Read the model definition and answer for the solid it produces. Units are mm, in the model's axes. A direction names the side the tool comes from. Coordinates: 2 decimals unless noted, no trailing zeros. Write each loop counter-clockwise with the first axis right and the second up, starting at its lowest first coordinate (ties: lowest second). Pieces come first, ordered by that corner, then holes.
(1) The part is cut by section B-B, the plane z = 5. State how many separate pieces and enclosed holes the cut face has, and give its area (3 significant figures).
(2) Straight lines are drawn through the part: line 1 along X through (y, z) = (12.7, 4.4); line 2 along Y through (x, z) = (12.7, 4.15); line 3 along X through (y, z) = (53, 1.75). For each, find the intervals that lie inside material, in ascending order.
(3) The part is cut by section C-C, the plane y = 80. Determine the outline of the cut face in (x, z), and give its area (3 significant figures).
(4) Which of the six approach directions +Z, -Z, +X, -X, +Y, -Y give full straight-line access (tool end or side, diameter ignored) to faces 4 (the flat face through (0, 50, 3)), 5 (the flat face through (38, 38, 3.175))?
(5) The part is cut by section A-A, the plane x = 12.7. Determine the outline of the cut face in (y, z) (3 decimals).
(6) Determine the mould class of faces 1 (the flat face through (5, 47, 0)), 2 (the flat face through (25, 0, 3)), 3 (the flat face through (13, 63, 3.175)) for opening direction Y: pulls with the +Y half, pulls with the -Y half, needs draft (parallel to the pull), parting line crosses it, or undercut.
(7) Given pin 1 (4 mm diameter, centred on x = 12.5, y = 13, fed in from +Z) (3 decimals); pin 2 (11.5 mm diameter, centred on x = 12.7, y = 12.7, fed in from -Z), each flat-ended and moving along its own axis, determine where each tip first touches the part or whether it passes through.
(8) The part is cut by section D-D, the plane x = 30. Determine the outline of the cut face in (y, z), and give its area (3 significant figures).
```python
from build123d import *

# Parameters (mm, degrees)
SKETCH1_W           = 50.8
SKETCH1_H           = 101.6
BOSS_EXTRUDE1_DEPTH = 6.35
SKETCH3_R           = 6.35
SKETCH3_R_2         = 2.54
CUT_EXTRUDE2_DEPTH  = 3.175
SKETCH4_W           = 38.1
SKETCH4_H           = 88.9
CUT_EXTRUDE3_DEPTH  = 2.54
CUT_EXTRUDE4_REACH  = 115.77
SKETCH5_W           = 38.1
SKETCH5_H           = 1.27


with BuildPart() as part:
    # Sketch1 → Boss-Extrude1 (new body)
    with BuildSketch(Plane.XY):
        with Locations((25.4, 50.8)):
            Rectangle(SKETCH1_W, SKETCH1_H)
    extrude(amount=BOSS_EXTRUDE1_DEPTH)

    # Sketch3 → Cut-Extrude2 (cut)
    with BuildSketch(Plane.XY.offset(6.35)):
        with Locations((12.7, 139.7)):
            Circle(SKETCH3_R)
        with Locations((38.1, 139.7)):
            Circle(SKETCH3_R)
        with Locations((63.5, 139.7)):
            Circle(SKETCH3_R_2)
        with Locations((88.9, 139.7)):
            Circle(SKETCH3_R_2)
        with Locations((88.9, 114.3)):
            Circle(SKETCH3_R_2)
        with Locations((63.5, 114.3)):
            Circle(SKETCH3_R_2)
        with Locations((38.1, 114.3)):
            Circle(SKETCH3_R)
        with Locations((12.7, 114.3)):
            Circle(SKETCH3_R)
        with Locations((88.9, 88.9)):
            Circle(SKETCH3_R_2)
        with Locations((63.5, 88.9)):
            Circle(SKETCH3_R_2)
        with Locations((38.1, 88.9)):
            Circle(SKETCH3_R)
        with Locations((12.7, 88.9)):
            Circle(SKETCH3_R)
        with Locations((88.9, 63.5)):
            Circle(SKETCH3_R_2)
        with Locations((63.5, 63.5)):
            Circle(SKETCH3_R_2)
        with Locations(Location((38.1, 63.5, 0), (0, 0, 180))):
            Circle(SKETCH3_R)
        with Locations(Location((12.7, 63.5, 0), (0, 0, 180))):
            Circle(SKETCH3_R)
        with Locations((88.9, 38.1)):
            Circle(SKETCH3_R_2)
        with Locations((63.5, 38.1)):
            Circle(SKETCH3_R_2)
        with Locations((38.1, 38.1)):
            Circle(SKETCH3_R)
        with Locations((12.7, 38.1)):
            Circle(SKETCH3_R)
        with Locations((88.9, 12.7)):
            Circle(SKETCH3_R_2)
        with Locations((63.5, 12.7)):
            Circle(SKETCH3_R_2)
        with Locations(Location((38.1, 12.7, 0), (0, 0, 180))):
            Circle(SKETCH3_R)
        with Locations(Location((12.7, 12.7, 0), (0, 0, 180))):
            Circle(SKETCH3_R)
    extrude(amount=-CUT_EXTRUDE2_DEPTH, mode=Mode.SUBTRACT)

    # Sketch4 → Cut-Extrude3 (cut)
    with BuildSketch(Plane(origin=(0, 0, 0), x_dir=(-1, 0, 0), z_dir=(0, 0, -1))):
        with Locations((-25.4, 50.8)):
            Rectangle(SKETCH4_W, SKETCH4_H)
    extrude(amount=-CUT_EXTRUDE3_DEPTH, mode=Mode.SUBTRACT)

    # Sketch5 → Cut-Extrude4 (cut, up to next)
    with BuildSketch(Plane(origin=(0, 101.6, 0), x_dir=(1, 0, 0), z_dir=(0, 1, 0)), mode=Mode.PRIVATE) as cut_extrude4_sk1:
        with Locations((25.4, -1.905)):
            Rectangle(SKETCH5_W, SKETCH5_H)
    cut_extrude4_tool1 = extrude(cut_extrude4_sk1.sketch, amount=-CUT_EXTRUDE4_REACH, mode=Mode.PRIVATE) & part.part
    add(cut_extrude4_tool1.solids().sort_by_distance((25.4, 101.6, 1.905))[0], mode=Mode.SUBTRACT)


solid = part.part
```
Computed:
1. separate pieces: 1
1. enclosed holes: 8
1. area: 4,150 mm2
2. line 1: x = 0 to 6.35, 19.05 to 31.75, 44.45 to 50.8
2. line 2: y = 0 to 6.35, 19.05 to 31.75, 44.45 to 57.15, 69.85 to 82.55, 95.25 to 101.6
2. line 3: x = 0 to 6.35, 44.45 to 50.8
3. outline: (0, 0) - (6.35, 0) - (6.35, 2.54) - (44.45, 2.54) - (44.45, 0) - (50.8, 0) - (50.8, 6.35) - (0, 6.35) - close
3. area: 226 mm2
4. face 4: +Z, -Z, -X, +Y, -Y
4. face 5: +Z
5. outline: (0, 0) - (6.35, 0) - (6.35, 2.54) - (101.6, 2.54) - (101.6, 6.35) - (95.25, 6.35) - (95.25, 3.175) - (82.55, 3.175) - (82.55, 6.35) - (69.85, 6.35) - (69.85, 3.175) - (57.15, 3.175) - (57.15, 6.35) - (44.45, 6.35) - (44.45, 3.175) - (31.75, 3.175) - (31.75, 6.35) - (19.05, 6.35) - (19.05, 3.175) - (6.35, 3.175) - (6.35, 6.35) - (0, 6.35) - close; (95.25, 0) - (101.6, 0) - (101.6, 1.27) - (95.25, 1.27) - close
6. face 1: needs draft
6. face 2: pulls with the -Y half
6. face 3: undercut
7. pin 1: stops at z = 3.175
7. pin 2: stops at z = 2.54
8. outline: (0, 0) - (6.35, 0) - (6.35, 2.54) - (101.6, 2.54) - (101.6, 6.35) - (0, 6.35) - close; (95.25, 0) - (101.6, 0) - (101.6, 1.27) - (95.25, 1.27) - close
8. area: 411 mm2
